```python
from build123d import *

# Parameters (mm, degrees)
SKETCH_2_R                   = 1.5
EXTRUDE_1_DEPTH              = 20
CUT_EXTRUDE_START            = 3
SKETCH_4_R                   = 32
CUT_EXTRUDE_1_DEPTH          = 15
SKETCH_6_R                   = 2
SKETCH_6_R_2                 = 4
CUT_EXTRUDE_2_DEPTH          = 106.996462205
SKETCH_8_W                   = 15
SKETCH_8_H                   = 45
EXTRUDE_3_DEPTH              = 10
HOLE_WIZARD_M5_1_D           = 5.5
HOLE_WIZARD_M5_1_CBORE_D     = 11
HOLE_WIZARD_M5_1_CBORE_DEPTH = 0.5
FILLET_1_R                   = 1


with BuildPart() as part:
    # 草图2 → 凸台-拉伸1 (new body)
    with BuildSketch(Plane(origin=(0, 0, 0), x_dir=(1, 0, 0), z_dir=(0, 1, 0))):
        with BuildLine():
            Line((0, 22.5), (100, 22.5))
            Line((100, 22.5), (100, -22.5))
            Line((100, -22.5), (0, -22.5))
            ThreePointArc((0, -22.5), (-22.5, 0), (0, 22.5))
        make_face()
        with Locations(Location((-15, 0, 0), (0, 0, 270))):
            Circle(SKETCH_2_R, mode=Mode.SUBTRACT)
        with Locations(Location((0, 15, 0), (0, 0, 270))):
            Circle(SKETCH_2_R, mode=Mode.SUBTRACT)
        with Locations(Location((15, 0, 0), (0, 0, 270))):
            Circle(SKETCH_2_R, mode=Mode.SUBTRACT)
        with Locations(Location((0, -15, 0), (0, 0, 270))):
            Circle(SKETCH_2_R, mode=Mode.SUBTRACT)
    extrude(amount=EXTRUDE_1_DEPTH)

    # 草图4 → 切除-拉伸1 (cut)
    with BuildSketch(Plane(origin=(0, 0, 0), x_dir=(1, 0, 0), z_dir=(0, 1, 0)).offset(CUT_EXTRUDE_START)):
        Circle(SKETCH_4_R)
    extrude(amount=CUT_EXTRUDE_1_DEPTH, mode=Mode.SUBTRACT)

    # 草图5 → 旋转1 (revolve)
    with BuildSketch(Plane.XY, mode=Mode.PRIVATE) as revolve_1_sk:
        Polygon((0, 20), (-20, 20), (-20, 21), (-17.5, 21), (-17.5, 27), (0, 27), align=None)
    revolve(revolve_1_sk.sketch.rotate(Axis((0, 42.215312946, 0), (0, -1, 0)), 270), axis=Axis((0, 42.215312946, 0), (0, -1, 0)))

    # 草图6 → 切除-拉伸2 (cut, through all)
    with BuildSketch(Plane(origin=(0, 0, 0), x_dir=(1, 0, 0), z_dir=(0, 1, 0))):
        with Locations(Location((0, 15, 0), (0, 0, 270))):
            Circle(SKETCH_6_R)
        with Locations(Location((15, 0, 0), (0, 0, 270))):
            Circle(SKETCH_6_R)
        with Locations(Location((0, -15, 0), (0, 0, 270))):
            Circle(SKETCH_6_R)
        with Locations(Location((-15, 0, 0), (0, 0, 270))):
            Circle(SKETCH_6_R)
        with Locations(Location((0, 0, 0), (0, 0, 270))):
            Circle(SKETCH_6_R_2)
    extrude(amount=CUT_EXTRUDE_2_DEPTH, mode=Mode.SUBTRACT)

    # 草图8 → 凸台-拉伸3 (add)
    with BuildSketch(Plane(origin=(0, 0, 0), x_dir=(1, 0, 0), z_dir=(0, 1, 0))):
        with Locations((107.5, 0)):
            Rectangle(SKETCH_8_W, SKETCH_8_H)
    extrude(amount=EXTRUDE_3_DEPTH)

    # M5 六角头螺栓的柱形沉头孔1 (through all)
    with Locations(Plane(origin=(0, 0, 0), x_dir=(-1, 0, 0), z_dir=(0, -1, 0))):
        with Locations((-107.5, -14), (-107.5, 0), (-107.5, 14)):
            CounterBoreHole(HOLE_WIZARD_M5_1_D / 2, HOLE_WIZARD_M5_1_CBORE_D / 2, HOLE_WIZARD_M5_1_CBORE_DEPTH)

    # 圆角1
    fillet_1_edges = [part.edges().sort_by_distance(p)[0] for p in [
        (32, 3, 0),
        (32, 18, 0),
    ]]
    fillet(fillet_1_edges, radius=FILLET_1_R)


solid = part.part
```
Can you work these out from the model? Positions are in its coordinate system, mm. A direction names the side the tool comes from. Coordinates: 2 decimals unless noted, no trailing zeros. Write each loop counter-clockwise with the first axis right and the second up, starting at its lowest first coordinate (ties: lowest second). Pieces come first, ordered by that corner, then holes. Notation, with made-up numbers: M 3,-3.75 L 39,-3.75 A23 cw 39,23.25 Z; hole C 39,78.5 d2. An arc over 180 degrees is marked long. Write item = value, one per line. Start each with the question number.
Q1. I'm going to push flat-ended pins straight in: pin 1 (2.5 mm diameter, centred on x = 0, z = 15, fed in from -Y); pin 2 (8 mm diameter, centred on x = 35, z = -2.5, fed in from +Y); pin 3 (17.5 mm diameter, centred on x = 107.5, z = 14, fed in from -Y); pin 4 (7 mm diameter, centred on x = 107.5, z = 0, fed in from -Y). Where does each tip first touch, or does it pass through?
Q2. If we section it at C-C, the plane y = 13: Write out the boundary of the cut face in (x, z), then the cut area to 3 significant figures.
Q3. On a 3-axis mill with a long thin cutter (end or side, diameter ignored), from which of +Z, -Z, +X, -X, +Y, -Y can I reach the whole of each face in a straight line? I mean faces 4 (the face through (19.524, 20.507, -4.336)), 5 (the face through (69, 10, -22.5)), 6 (the face through (104.753, 5.316, -0.121)), 7 (the face through (32, 10, 0)), 8 (the face through (112.995, 0.246, -0.242)). Say none if no direction works.
Q4. If we section it at B-B, the plane x = -15: Write out the boundary of the cut face in (y, z).
Q5. Thinking about a two-plate mould opening in Y: for faces 1 (the face through (106, 0.5, 11)), 2 (the face through (4, 3, -5)), 3 (the face through (112.995, 0.246, -14.242)), which applies, released by +Y, released by -Y, zero draft, split by the parting line, or undercut?
Q6. If we section it at A-A, the plane y = 23.5: Write out the boundary of the cut face in (x, z).
Q7. If we section it at D-D, the plane x = 51: Write out the boundary of the cut face in (y, z).
Q8. If I drill on L1, parallel to Z at x = 0, y = 1.75; L2, parallel to Z at x = 107.5, y = 0.45; L3, parallel to X at y = 22, z = 0, over which ranges is the centre line in solid material (lowest first)? Write a range as [from, to].
Check sheet entries:
q1.pin_1 = through
q1.pin_2 = 20
q1.pin_3 = 0
q1.pin_4 = 0.5
q2.outline = M 22.75,-22.5 L 100,-22.5 L 100,22.5 L 22.75,22.5 A32 cw Z
q2.area = 3,190 mm²
q3.face_4 = +Y
q3.face_5 = -Z, +X, -X, +Y, -Y
q3.face_6 = +Y, -Y
q3.face_7 = -X
q3.face_8 = -Y
q4.outline = M 0,-16.77 L 3,-16.77 L 3,-2 L 0,-2 Z; M 0,2 L 3,2 L 3,16.77 L 0,16.77 Z; M 18,-16.77 L 20,-16.77 L 20,-13.23 L 21,-13.23 L 21,-9.01 L 27,-9.01 L 27,-2 L 18,-2 Z; M 18,2 L 27,2 L 27,9.01 L 21,9.01 L 21,13.23 L 20,13.23 L 20,16.77 L 18,16.77 Z
q5.face_1 = released by -Y
q5.face_2 = undercut
q5.face_3 = zero draft
q6.outline = C 0,0 d35; hole C -15,0 d4; hole C 0,0 d8; hole C 0,-15 d4; hole C 0,15 d4; hole C 15,0 d4
q7.outline = M 0,-22.5 L 20,-22.5 L 20,22.5 L 0,22.5 Z
q8.L1 = [-22.5, -17], [-13, -4], [4, 13], [17, 22.5]
q8.L2 = [-22.5, -19.5], [-8.5, -5.5], [5.5, 8.5], [19.5, 22.5]
q8.L3 = [-17.5, -17], [-13, -4], [4, 13], [17, 17.5]
